Here's how the part is built. I have some questions about the finished solid (model axes, mm). Face numbers are marked on the shaded views. Coordinates: 2 decimals unless noted, no trailing zeros. Write each loop counter-clockwise with the first axis right and the second up, starting at its lowest first coordinate (ties: lowest second). Pieces come first, ordered by that corner, then holes. Notation, with made-up numbers: (-11.5, -29.5) -> (-7.5, -29.5) arc R16 cw to (-7.5, 0.5) -> close; hole circle Ø6 at (1.5, 15.5). An arc over 180 degrees is marked (long way). Put each result on its own line as item: value.
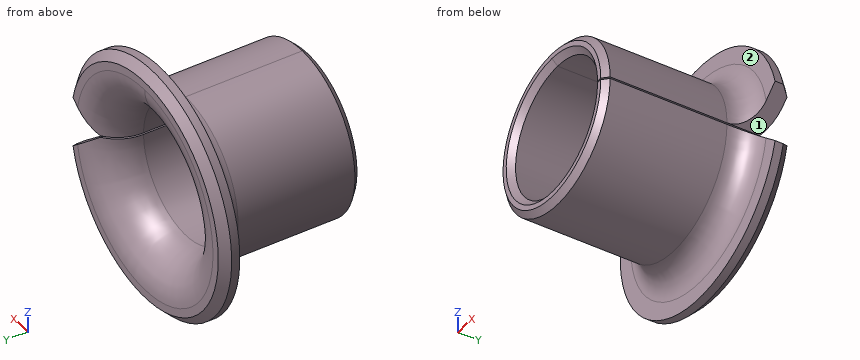
```python
from build123d import *

# Parameters (mm, degrees)
F2_SIZE  = 0.35
F3_R     = 1.5
F4_R     = 2.5
F5_SIZE  = 0.5
F7_DEPTH = 10.0010001


with BuildPart() as f1:
    # F0 (on Right) → F1 (revolve)
    with BuildSketch(Plane.YZ):
        Polygon((5, 4), (5, 7.5), (4, 7.5), (4, 5), (-5, 5), (-5, 4), align=None)
    revolve(axis=Axis((0, 0, 0), (0, 1, 0)))

    # F2
    f2_edges = [f1.edges().sort_by_distance(p)[0] for p in [
        (0, -5, -5),
        (0, -5, -4),
    ]]
    chamfer(f2_edges, length=F2_SIZE)

    # F3
    f3_edges = [f1.edges().sort_by_distance(p)[0] for p in [
        (0, 4, -5),
    ]]
    fillet(f3_edges, radius=F3_R)

    # F4
    f4_edges = [f1.edges().sort_by_distance(p)[0] for p in [
        (0, 5, -4),
    ]]
    fillet(f4_edges, radius=F4_R)

    # F5
    f5_edges = [f1.edges().sort_by_distance(p)[0] for p in [
        (0, 5, -7.5),
    ]]
    chamfer(f5_edges, length=F5_SIZE)

    # F6 (on face) → F7 (cut, through all)
    with BuildSketch(Plane.XZ.offset(5)):
        with BuildLine():
            Line((4.9997499937, 0.05), (4.649731175, 0.05))
            ThreePointArc((4.649731175, 0.05), (4.6499327933, 0.0250003613), (4.65, 0))
            ThreePointArc((4.65, 0), (4.6499327933, -0.0250003613), (4.649731175, -0.05))
            Line((4.649731175, -0.05), (4.9997499937, -0.05))
            Line((4.9997499937, -0.05), (8, -2.5675086737))
            Line((8, -2.5675086737), (8, 2.5675086737))
            Line((8, 2.5675086737), (4.9997499937, 0.05))
        make_face()
        with BuildLine():
            Line((4.3497126342, 0.05), (3.9996874878, 0.05))
            Line((3.9996874878, 0.05), (3.9996874878, -0.05))
            Line((3.9996874878, -0.05), (4.3497126342, -0.05))
            ThreePointArc((4.3497126342, -0.05), (4.349928158, -0.0250004129), (4.35, 0))
            ThreePointArc((4.35, 0), (4.349928158, 0.0250004129), (4.3497126342, 0.05))
        make_face()
        with BuildLine():
            Line((4.649731175, 0.05), (4.3497126342, 0.05))
            ThreePointArc((4.3497126342, 0.05), (4.349928158, 0.0250004129), (4.35, 0))
            ThreePointArc((4.35, 0), (4.349928158, -0.0250004129), (4.3497126342, -0.05))
            Line((4.3497126342, -0.05), (4.649731175, -0.05))
            ThreePointArc((4.649731175, -0.05), (4.6499327933, -0.0250003613), (4.65, 0))
            ThreePointArc((4.65, 0), (4.6499327933, 0.0250003613), (4.649731175, 0.05))
        make_face()
    extrude(amount=-F7_DEPTH, mode=Mode.SUBTRACT)


solid = f1.part
```
Item 1: For P1, Ø3, axis at y = -3, z = -1.5, coming from the +X side; P2, Ø6, axis at x = -1, y = -1.5, coming from the +Z side; P3, Ø1.1, axis at x = 4.5, y = 1.5, coming from the -Z side; P4, Ø6.5, axis at x = 0, z = 0, coming from the +Y side, each with a flat end and sliding along its axis, tell me the tip position at first contact or that it passes through.
Output:
P1: stops at x = 5
P2: stops at z = 5
P3: stops at z = -3.07
P4: passes through
Item 2: Imagine slicing it at A-A on y = 3.75. Write out the boundary of the cut face in (x, z).
Output:
outline: (4.33, -0.05) arc R4.33 cw (long way) to (4.33, 0.05) -> (5, 0.05) -> (5.64, 0.59) arc R5.67 ccw (long way) to (5.64, -0.59) -> (5, -0.05) -> close
Item 3: Imagine slicing it at B-B on y = -2.5. Write out the boundary of the cut face in (x, z).
Output:
outline: (4, -0.05) arc R4 cw (long way) to (4, 0.05) -> (5, 0.05) arc R5 ccw (long way) to (5, -0.05) -> close
Item 4: Please list where these lines run through material, in increasing order: line 1 along X through (y, z) = (-0.75, 0); line 2 along Z through (x, y) = (0, 0.5); line 3 along X through (y, z) = (-2, 1.5). Write a range as from..to.
Output:
line 1: x = -5..-4
line 2: z = -5..-4, 4..5
line 3: x = -4.77..-3.71, 3.71..4.77
Item 5: If we mould it in two halves opening along Z, with no side actions, what happens to the marked faces 1 and 2? For each: released by +Z, released by -Z, zero draft, split by the parting line, or undercut.
Output:
face 1: undercut
face 2: zero draft
